from build123d import *

# Parameters (mm, degrees)
SKETCH_R        = 27
SKETCH_R_2      = 10
PAD_DEPTH       = 2
SKETCH001_R     = 2
POCKET_DEPTH    = 2.001
SKETCH002_R     = 19.8
SKETCH002_R_2   = 18.3
PAD001_DEPTH    = 5
POCKET001_DEPTH = 5
SKETCH004_R     = 2
POCKET002_DEPTH = 2.001
CHAMFER_SIZE    = 0.7


with BuildPart() as part:
    # Sketch → Pad (new body)
    with BuildSketch(Plane.XY):
        Circle(SKETCH_R)
        Circle(SKETCH_R_2, mode=Mode.SUBTRACT)
    extrude(amount=PAD_DEPTH)

    # Sketch001 (on Face4 of Pad) → Pocket (cut, through all)
    with BuildSketch(Plane.XY.offset(2)):
        with Locations((0, 14)):
            Circle(SKETCH001_R)
        with Locations((14, 0)):
            Circle(SKETCH001_R)
        with Locations((0, -14)):
            Circle(SKETCH001_R)
        with Locations((-14, 0)):
            Circle(SKETCH001_R)
    extrude(amount=-POCKET_DEPTH, mode=Mode.SUBTRACT)

    # Sketch002 (on Face3 of Pocket) → Pad001 (join)
    with BuildSketch(Plane.XY.offset(2)):
        Circle(SKETCH002_R)
        Circle(SKETCH002_R_2, mode=Mode.SUBTRACT)
    extrude(amount=PAD001_DEPTH)

    # Sketch003 (on Face3 of Pad001) → Pocket001 (cut)
    with BuildSketch(Plane.XY.offset(2)):
        Polygon((-49.376067, 10), (-10, 10), (-10, 45.075482), (10, 45.075482), (10, 10), (49.376067, 10), (49.376067, -10), (10, -10), (10, -45.075482), (-10, -45.075482), (-10, -10), (-49.376067, -10), align=None)
    extrude(amount=POCKET001_DEPTH, mode=Mode.SUBTRACT)

    # Sketch004 (on Face24 of Pocket001) → Pocket002 (cut, through all)
    with BuildSketch(Plane.XY.offset(2)):
        with Locations((-21.5, 0)):
            Circle(SKETCH004_R)
        with Locations((21.5, 0)):
            Circle(SKETCH004_R)
    extrude(amount=-POCKET002_DEPTH, mode=Mode.SUBTRACT)

    # Chamfer
    chamfer_edges = [part.edges().sort_by_distance(p)[0] for p in [
        (14.000714, -14.000714, 7),
        (-14.000714, -14.000714, 7),
        (-14.000714, 14.000714, 7),
        (14.000714, 14.000714, 7),
    ]]
    chamfer(chamfer_edges, length=CHAMFER_SIZE)


solid = part.part
Could you check a few things on this model? Use its own coordinates, in mm. A direction names the side the tool comes from. Give positions to 0.01 mm unless a question says otherwise; leave off trailing zeros. Order: outer loops, then holes, each group sorted by start corner. A loop starts at its lowest first (then second) coordinate and runs counter-clockwise, first axis right, second up.
1. Suppose I cut it at D-D (y = 6). Write out the boundary of the cut face in (x, z), plus the area to 3 significant figures.
Answers below:
outline: (-26.32, 0) - (-8, 0) - (-8, 2) - (-26.32, 2) - close; (8, 0) - (26.32, 0) - (26.32, 2) - (8, 2) - close
area: 73.3 mm2
2. Which directions (+Z, -Z, +X, -X, +Y, -Y) give clear straight access to the entire face, cutting with the end or side of a thin tool? Please do faces 1 (the flat face through (16, -10, 4)), 2 (the cylindrical face through (-14, -14, 4)), 3 (the flat face through (-10, 16, 4)).
Answers below:
face 1: +Z, +X, -X
face 2: +Z, -X, -Y
face 3: +Z, +Y, -Y
3. I need wall thicknesses on L1, parallel to Y at x = 0, z = 1; L2, parallel to Z at x = -21, y = 12; L3, parallel to Y at x = -10.5, z = 2.25. Which ranges of each line are inside material? Lowest first, please.
Answers below:
L1: y = -27 to -16, -12 to -10, 10 to 12, 16 to 27
L2: z = 0 to 2
L3: y = -16.79 to -14.99, 14.99 to 16.79
4. Suppose I cut it at C-C (z = 3.75). Write out the boundary of the cut face in (x, y).
Answers below:
outline: (-17.09, -10) arc R19.8 ccw to (-10, -17.09) - (-10, -15.33) arc R18.3 cw to (-15.33, -10) - close; (-17.09, 10) - (-15.33, 10) arc R18.3 cw to (-10, 15.33) - (-10, 17.09) arc R19.8 ccw to start; (10, -17.09) arc R19.8 ccw to (17.09, -10) - (15.33, -10) arc R18.3 cw to (10, -15.33) - close; (10, 15.33) arc R18.3 cw to (15.33, 10) - (17.09, 10) arc R19.8 ccw to (10, 17.09) - close
5. Thinking about a two-plate mould opening in Y: for faces 4 (the conical face through (-13.65, 13.74, 6.73)), 5 (the cylindrical face through (12.9, -12.98, 4.46)), 6 (the conical face through (-13.74, -13.65, 6.73)), 7 (the cylindrical face through (-15.6, -1.2, 1)), which applies, +Y half, -Y half, draft (parallel to the pull), parting line (faces both ways), or undercut?
Answers below:
face 4: +Y half
face 5: undercut
face 6: -Y half
face 7: undercut
6. Suppose I cut it at B-B (y = 0). Write out the boundary of the cut face in (x, z), plus the area to 3 significant figures.
Answers below:
outline: (-27, 0) - (-23.5, 0) - (-23.5, 2) - (-27, 2) - close; (-19.5, 0) - (-16, 0) - (-16, 2) - (-19.5, 2) - close; (-12, 0) - (-10, 0) - (-10, 2) - (-12, 2) - close; (10, 0) - (12, 0) - (12, 2) - (10, 2) - close; (16, 0) - (19.5, 0) - (19.5, 2) - (16, 2) - close; (23.5, 0) - (27, 0) - (27, 2) - (23.5, 2) - close
area: 36.0 mm2
7. Suppose I cut it at A-A (x = 0). Write out the boundary of the cut face in (y, z), plus the area to 3 significant figures.
Answers below:
outline: (-27, 0) - (-16, 0) - (-16, 2) - (-27, 2) - close; (-12, 0) - (-10, 0) - (-10, 2) - (-12, 2) - close; (10, 0) - (12, 0) - (12, 2) - (10, 2) - close; (16, 0) - (27, 0) - (27, 2) - (16, 2) - close
area: 52.0 mm2
8. For pin 1 (3 mm diameter, centred on x = -10.5, y = -21, fed in from +Z); pin 2 (1.9 mm diameter, centred on x = -16, z = 5.5, fed in from -Y); pin 3 (0.5 mm diameter, centred on x = 16.5, z = 3.5, fed in from +Y); pin 4 (4.5 mm diameter, centred on x = 14, y = 0, fed in from -Z), each with a flat end and sliding along its axis, tell me the tip position at first contact or that it passes through.
Answers below:
pin 1: stops at z = 2
pin 2: stops at y = -12.87
pin 3: stops at y = 11.31
pin 4: stops at z = 0
